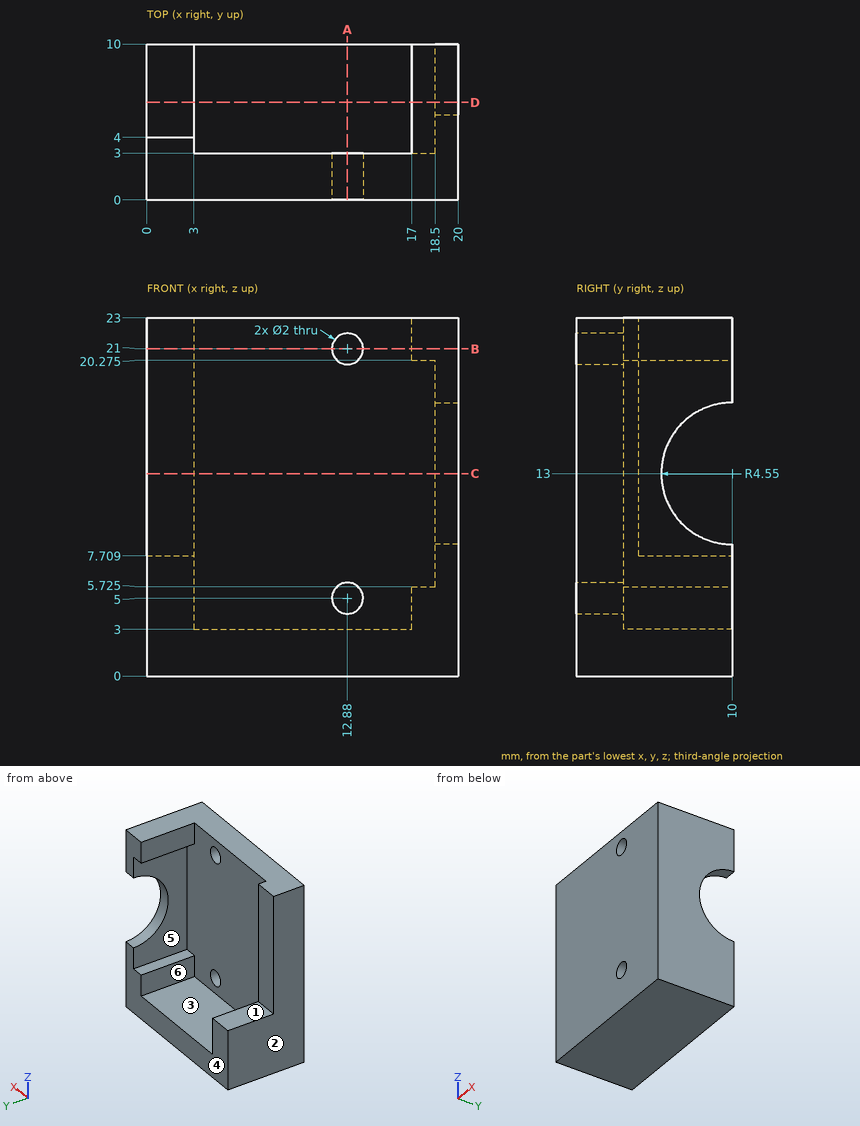
Print and shaded views of the part. All mm, measured from the part's lowest x, y and z. A direction names the side the tool comes from. Coordinates: 2 decimals unless noted, no trailing zeros. Order: outer loops, then holes, each group sorted by start corner. A loop starts at its lowest first (then second) coordinate and runs counter-clockwise, first axis right, second up. Notation, with made-up numbers: (62.5, -5) -> (90.5, -5) arc R17 cw to (90.5, 6) -> close; hole circle Ø11 at (1.25, 47). An arc over 180 degrees is marked (long way). Use one line per item in the form item = value. Start each with the question number.
1) Drill centre lines: L1, parallel to X at y = 6.75, z = 3.5; L2, parallel to X at y = 1.9, z = 21; L3, parallel to Y at x = 8, z = 4.25. Where is each one in solid material? Low to high. Write a range as [from, to].
2) Tool access for the marked faces 4, 5 and 6: list every direction of +Z, -Z, +X, -X, +Y, -Y with a clear straight run to the whole face (end or side of a thin tool).
3) Band-saw the part on C-C on z = 13. Give the cut face in (x, y).
4) Band-saw the part on A-A on x = 12.88. Give the cut face in (y, z).
5) Band-saw the part on B-B on z = 21. Give the cut face in (x, y).
6) Band-saw the part on D-D on y = 6.25. Give the cut face in (x, z) (1 decimal).
7) Drop flat-ended pins along their axis: pin 1 (5.5 mm diameter, centred on x = 6.5, y = 6.5, fed in from +Z); pin 2 (1.4 mm diameter, centred on y = 5, z = 21.5, fed in from -X); pin 3 (8 mm diameter, centred on x = 10.5, z = 9, fed in from +Y). Give the stop position or say it passes through.
8) Pull direction X, two halves, no side cores. Call the marked faces 1, 2 and 3: +X half, -X half, draft (parallel to the pull), parting line (faces both ways), or undercut.
Entries:
q1.L1 = [0, 3], [17, 20]
q1.L2 = [0, 11.88], [13.88, 20]
q1.L3 = [0, 3]
q2.face_4 = +Z, -Z, +X, -X, +Y
q2.face_5 = +Y
q2.face_6 = +Z, +Y
q3.outline = (0, 0) -> (20, 0) -> (20, 5.45) -> (18.5, 5.45) -> (18.5, 3) -> (3, 3) -> (3, 4) -> (0, 4) -> close
q4.outline = (0, 0) -> (10, 0) -> (10, 3) -> (3, 3) -> (3, 4) -> (0, 4) -> close; (0, 6) -> (3, 6) -> (3, 20) -> (0, 20) -> close; (0, 22) -> (3, 22) -> (3, 23) -> (0, 23) -> close
q5.outline = (0, 0) -> (11.88, 0) -> (11.88, 3) -> (3, 3) -> (3, 4) -> (0, 4) -> close; (13.88, 0) -> (20, 0) -> (20, 10) -> (17, 10) -> (17, 3) -> (13.88, 3) -> close
q6.outline = (0, 0) -> (20, 0) -> (20, 10.4) -> (18.5, 10.4) -> (18.5, 5.7) -> (17, 5.7) -> (17, 3) -> (3, 3) -> (3, 7.7) -> (0, 7.7) -> close; (17, 20.3) -> (18.5, 20.3) -> (18.5, 15.6) -> (20, 15.6) -> (20, 23) -> (17, 23) -> close
q7.pin_1 = 3
q7.pin_2 = 17
q7.pin_3 = 3
q8.face_1 = draft
q8.face_2 = -X half
q8.face_3 = undercut
